Input: part model. Units: mm. Frame: model coordinates. Round coordinates to 2 decimals unless told otherwise and drop trailing zeros. Write each loop counter-clockwise with the first axis right and the second up, starting at its lowest first coordinate (ties: lowest second). Pieces come first, ordered by that corner, then holes. Notation, with made-up numbers: (73, 46) - (99, 46) arc R34 cw to (99, 76) - close; hole circle Ø6 at (57, -32). An arc over 180 degrees is marked (long way). One line per item, written item: value. Start each with the question number.
```python
from build123d import *

# Parameters (mm, degrees)
F0_W      = 254
F0_H      = 170
F0_R      = 2.2742272187
F1_DEPTH  = 3
F2_W      = 254
F2_H      = 170
F2_W_2    = 238
F2_H_2    = 150
F3_DEPTH  = 10
F4_R      = 3
F5_R      = 1.5
F6_DEPTH  = 25
F7_W      = 26.6
F7_H      = 65
F7_W_2    = 65
F7_H_2    = 26
F8_DEPTH  = 1
F9_W      = 10
F9_H      = 10
F10_DEPTH = 25


# Not quite as in the source:
# - a feature names something its author has since deleted; it is built from what else it names


with BuildPart() as f1:
    # F0 (on Top) → F1 (new body)
    with BuildSketch(Plane.XY):
        Rectangle(F0_W, F0_H)
        with Locations((-100, -50)):
            Circle(F0_R, mode=Mode.SUBTRACT)
        with Locations((100, -50)):
            Circle(F0_R, mode=Mode.SUBTRACT)
        with Locations((-100, 50)):
            Circle(F0_R, mode=Mode.SUBTRACT)
        with Locations((100, 50)):
            Circle(F0_R, mode=Mode.SUBTRACT)
    extrude(amount=F1_DEPTH)

    # F2 (on face) → F3 (join)
    with BuildSketch(Plane.XY.offset(3)):
        Rectangle(F2_W, F2_H)
        Rectangle(F2_W_2, F2_H_2, mode=Mode.SUBTRACT)
    extrude(amount=-F3_DEPTH)

    # F4
    f4_edges = [f1.edges().sort_by_distance(p)[0] for p in [
        (-127, 0, -7),
        (-119, 0, -7),
        (0, 75, -7),
        (0, 85, -7),
        (119, 0, -7),
        (127, 0, -7),
        (0, -75, -7),
        (0, -85, -7),
    ]]
    fillet(f4_edges, radius=F4_R)

    # F5 (on face) → F6 (cut)
    with BuildSketch(Plane.XY.offset(3)):
        with Locations((-34.4810113311, -23.1507848948)):
            Circle(F5_R)
        with Locations((-34.4810113311, 26.8492151052)):
            Circle(F5_R)
        with Locations((37.5189886689, -23.1507848948)):
            Circle(F5_R)
        with Locations((37.5189886689, 26.8492151052)):
            Circle(F5_R)
    extrude(amount=-F6_DEPTH, mode=Mode.SUBTRACT)

    # F7 (on face) → F8 (join)
    with BuildSketch(Plane.XY.offset(3)):
        with Locations((-90, 0)):
            Rectangle(F7_W, F7_H)
        with Locations((0, 51.8365384532)):
            Rectangle(F7_W_2, F7_H_2)
        with Locations((0, -51.8365384532)):
            Rectangle(F7_W_2, F7_H_2)
        with Locations((90, 0)):
            Rectangle(F7_W, F7_H)
    extrude(amount=F8_DEPTH)

    # F9 (on face) → F10 (cut)
    with BuildSketch(Plane.XY.offset(3)):
        with Locations((-47.5, 51.8365384532)):
            Rectangle(F9_W, F9_H)
        with Locations((90, 42.4970947206)):
            Rectangle(F9_W, F9_H)
        with Locations((41.3667224348, -51.8365384532)):
            Rectangle(F9_W, F9_H)
        with Locations((-90, -42.1905592084)):
            Rectangle(F9_W, F9_H)
    extrude(amount=-F10_DEPTH, mode=Mode.SUBTRACT)


solid = f1.part
```
Q1. Cut plane A-A, the plane x = -109. Output: boundary loops of the cut face in (y, z), and give its area (3 significant figures).
Q2. Material intervals for probe 1 along Y at (x, z) = (-100, 1.8); probe 2 along X at (y, z) = (52, -3); probe 3 along Y at (x, z) = (-99.5, -2), sorted ascending. Write a range as from..to.
Q3. Contact query for flat-ended pins moving along their axis: pin 1 Ø0.8 at (x, z) = (-5.5, 3.5) entering from +Y; pin 2 Ø2 at (x, z) = (46, -6) entering from +Y; pin 3 Ø0.5 at (y, z) = (6.5, 3.5) entering from +X. Output: stop coordinate, or through.
Q4. Pull-direction query (Y, two-part tool) for faces 1 (the flat face through (-2, -85, 0)), 2 (the flat face through (-2, 1, 0)), 3 (the flat face through (90, 0, 4)); classes: pulls with the +Y half, pulls with the -Y half, needs draft (parallel to the pull), parting line crosses it, or undercut.
A:
1. outline: (-85, -4) arc R3 ccw to (-82, -7) - (-78, -7) arc R3 ccw to (-75, -4) - (-75, 0) - (75, 0) - (75, -4) arc R3 ccw to (78, -7) - (82, -7) arc R3 ccw to (85, -4) - (85, 3) - (-85, 3) - close
1. area: 642 mm²
2. probe 1: y = -85..-52.27, -47.73..47.73, 52.27..85
2. probe 2: x = -127..-119, 119..127
2. probe 3: y = -85..-75, 75..85
3. pin 1: stops at y = 64.84
3. pin 2: stops at y = 84.83
3. pin 3: stops at x = 103.3
4. face 1: pulls with the -Y half
4. face 2: undercut
4. face 3: needs draft
